Part model, mm, in its own coordinate system. Round coordinates to 2 decimals unless told otherwise and drop trailing zeros. Write each loop counter-clockwise with the first axis right and the second up, starting at its lowest first coordinate (ties: lowest second). Pieces come first, ordered by that corner, then holes.
```python
from build123d import *

# Parameters (mm, degrees)
F1_DEPTH = 1.5875


with BuildPart() as f1:
    # F0 (on Top) → F1 (new body)
    with BuildSketch(Plane.XY):
        with BuildLine():
            ThreePointArc((0, 74.0791), (4.490128, 72.219228), (6.35, 67.7291))
            Line((6.35, 67.7291), (12.7, 67.7291))
            ThreePointArc((12.7, 67.7291), (8.980256, 76.709356), (0, 80.4291))
            Line((0, 80.4291), (0, 74.0791))
        make_face()
        with BuildLine():
            Line((12.7, 67.7291), (6.35, 67.7291))
            ThreePointArc((6.35, 67.7291), (4.490128, 63.238972), (0, 61.3791))
            Line((0, 61.3791), (0, -61.3791))
            ThreePointArc((0, -61.3791), (4.490128, -63.238972), (6.35, -67.7291))
            Line((6.35, -67.7291), (12.7, -67.7291))
            Line((12.7, -67.7291), (12.7, 67.7291))
        make_face()
        with BuildLine():
            ThreePointArc((-6.35, 67.7291), (-4.490128, 72.219228), (0, 74.0791))
            Line((0, 74.0791), (0, 80.4291))
            ThreePointArc((0, 80.4291), (-8.980256, 76.709356), (-12.7, 67.7291))
            Line((-12.7, 67.7291), (-6.35, 67.7291))
        make_face()
        with BuildLine():
            Line((0, -61.3791), (0, 61.3791))
            ThreePointArc((0, 61.3791), (-4.490128, 63.238972), (-6.35, 67.7291))
            Line((-6.35, 67.7291), (-12.7, 67.7291))
            Line((-12.7, 67.7291), (-12.7, -67.7291))
            Line((-12.7, -67.7291), (-6.35, -67.7291))
            ThreePointArc((-6.35, -67.7291), (-4.490128, -63.238972), (0, -61.3791))
        make_face()
        with BuildLine():
            ThreePointArc((0, -80.4291), (8.980256, -76.709356), (12.7, -67.7291))
            Line((12.7, -67.7291), (6.35, -67.7291))
            ThreePointArc((6.35, -67.7291), (4.490128, -72.219228), (0, -74.0791))
            Line((0, -74.0791), (0, -80.4291))
        make_face()
        with BuildLine():
            ThreePointArc((-12.7, -67.7291), (-8.980256, -76.709356), (0, -80.4291))
            Line((0, -80.4291), (0, -74.0791))
            ThreePointArc((0, -74.0791), (-4.490128, -72.219228), (-6.35, -67.7291))
            Line((-6.35, -67.7291), (-12.7, -67.7291))
        make_face()
    extrude(amount=F1_DEPTH)


solid = f1.part
```
Q1. Cut at D-D on x = 2.5. Write the cut outline in (y, z), plus the area to 3 significant figures.
Values follow:
outline: (-80.18, 0) - (-73.57, 0) - (-73.57, 1.59) - (-80.18, 1.59) - close; (-61.89, 0) - (61.89, 0) - (61.89, 1.59) - (-61.89, 1.59) - close; (73.57, 0) - (80.18, 0) - (80.18, 1.59) - (73.57, 1.59) - close
area: 218 mm2
Q2. Drop a flat-ended pin along its axis: pin 1 (8 mm diameter, centred on x = -1.5, y = -48.5, fed in from -Z). Give the stop position or say it passes through.
Values follow:
pin 1: stops at z = 0
Q3. Wall check: L1, parallel to Y at x = -0.5, z = 1.45; L2, parallel to Y at x = -1.25, z = 1.15; L3, parallel to X at y = -67.5, z = 0.1. Give the ranges that are in metal, low to high.
Values follow:
L1: y = -80.42 to -74.06, -61.4 to 61.4, 74.06 to 80.42
L2: y = -80.37 to -73.95, -61.5 to 61.5, 73.95 to 80.37
L3: x = -12.7 to -6.35, 6.35 to 12.7
Q4. Cut at A-A on x = -3.25. Write the cut outline in (y, z).
Values follow:
outline: (-80.01, 0) - (-73.18, 0) - (-73.18, 1.59) - (-80.01, 1.59) - close; (-62.27, 0) - (62.27, 0) - (62.27, 1.59) - (-62.27, 1.59) - close; (73.18, 0) - (80.01, 0) - (80.01, 1.59) - (73.18, 1.59) - close
Q5. Cut at B-B on z = 1. Write the cut outline in (x, y).
Values follow:
outline: (-12.7, -67.73) arc R12.7 ccw to (12.7, -67.73) - (12.7, 67.73) arc R12.7 ccw to (-12.7, 67.73) - close; hole circle Ø12.7 at (0, -67.73); hole circle Ø12.7 at (0, 67.73)
Q6. Cut at C-C on y = -64. Write the cut outline in (x, z).
Values follow:
outline: (-12.7, 0) - (-5.14, 0) - (-5.14, 1.59) - (-12.7, 1.59) - close; (5.14, 0) - (12.7, 0) - (12.7, 1.59) - (5.14, 1.59) - close
